Work out the finished part from the listing and answer in its coordinate system (mm). Face numbers are marked on the shaded views. A direction names the side the tool comes from. Round coordinates to 2 decimals unless told otherwise and drop trailing zeros. Order: outer loops, then holes, each group sorted by start corner. A loop starts at its lowest first (then second) coordinate and runs counter-clockwise, first axis right, second up. Notation, with made-up numbers: M 16,-12.75 L 46,-12.75 A21 cw 46,4.25 Z; hole C 18,-25.5 d10. An arc over 180 degrees is marked long. Return JSON: item names as keys, results as strings.
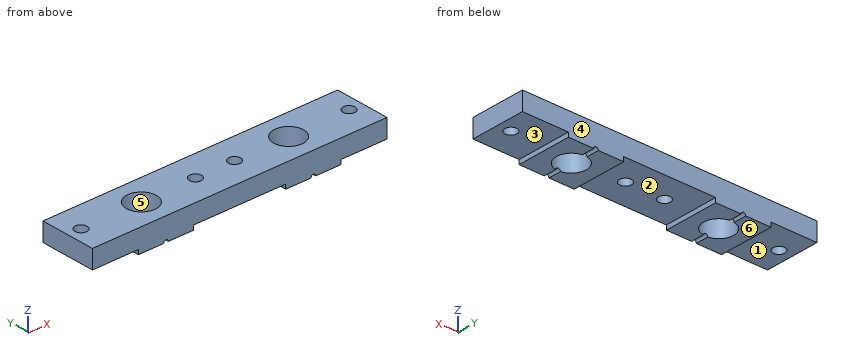
from build123d import *

# Parameters (mm, degrees)
SKETCH1_W                        = 101.6
SKETCH1_H                        = 19.05
EXTRUDE1_DEPTH                   = 7.9248
F_13_32_0_40625_DIAMETER_HOLE1_D = 10.31875
F_8_32_TAPPED_HOLE1_D            = 4.1656
SKETCH9_W                        = 31.75
SKETCH9_H                        = 19.05
SKETCH9_W_2                      = 15.875
EXTRUDE3_DEPTH                   = 1.524
F_1_16_0_0625_DIAMETER_HOLE1_D   = 1.5875


with BuildPart() as part:
    # Sketch1 → Extrude1 (new body)
    with BuildSketch(Plane.XY):
        Rectangle(SKETCH1_W, SKETCH1_H)
    extrude(amount=EXTRUDE1_DEPTH)

    # 13/32 (0.40625) Diameter Hole1 (through all)
    with Locations(Plane(origin=(0, 0, 0), x_dir=(-1, 0, 0), z_dir=(0, 0, -1))):
        with Locations((25.4, 0), (-25.4, 0)):
            Hole(F_13_32_0_40625_DIAMETER_HOLE1_D / 2)

    # #8-32 Tapped Hole1 (through all)
    with Locations(Plane.XY.offset(7.9248)):
        with Locations((-46.228, 0), (-6.731, 0), (6.731, 0), (46.228, 0)):
            Hole(F_8_32_TAPPED_HOLE1_D / 2)

    # Sketch9 → Extrude3 (cut)
    with BuildSketch(Plane(origin=(0, 0, 0), x_dir=(-1, 0, 0), z_dir=(0, 0, -1))):
        Rectangle(SKETCH9_W, SKETCH9_H)
        with Locations((-42.8625, 0)):
            Rectangle(SKETCH9_W_2, SKETCH9_H)
        with Locations((42.8625, 0)):
            Rectangle(SKETCH9_W_2, SKETCH9_H)
    extrude(amount=-EXTRUDE3_DEPTH, mode=Mode.SUBTRACT)

    # 1/16 (0.0625) Diameter Hole1 (through all)
    with Locations(Plane(origin=(0, 9.525, 0), x_dir=(-1, 0, 0), z_dir=(0, 1, 0))):
        with Locations((-25.4, 0), (25.4, 0)):
            Hole(F_1_16_0_0625_DIAMETER_HOLE1_D / 2)


solid = part.part
Item 1: Consider line 1 along Y through (x, z) = (-25, 1.75) (3 decimals); line 2 along X through (y, z) = (-3.5, 5); line 3 along X through (y, z) = (-4.5, 4.25). Determine where each line is inside the solid, lowest interval first. Write a range as [from, to].
Output:
{"line 1": "y = [-9.525, -5.144], [5.144, 9.525]", "line 2": "x = [-50.8, -29.19], [-21.61, 21.61], [29.19, 50.8]", "line 3": "x = [-50.8, -27.92], [-22.88, 22.88], [27.92, 50.8]"}
Item 2: Which of the six approach directions +Z, -Z, +X, -X, +Y, -Y give full straight-line access (tool end or side, diameter ignored) to the marked faces 1, 2 and 3?
Output:
{"face 1": "-Z, -X, +Y, -Y", "face 2": "-Z, +Y, -Y", "face 3": "-Z, +X, +Y, -Y"}
Item 3: Find section D-D (y = 3.5). Determine the outline of the cut face in (x, z) (3 decimals), plus the area to 3 significant figures.
Output:
{"outline": "M -50.8,1.524 L -34.925,1.524 L -34.925,0 L -29.191,0 L -29.191,7.925 L -50.8,7.925 Z; M -21.609,0 L -15.875,0 L -15.875,1.524 L 15.875,1.524 L 15.875,0 L 21.609,0 L 21.609,7.925 L -21.609,7.925 Z; M 29.191,0 L 34.925,0 L 34.925,1.524 L 50.8,1.524 L 50.8,7.925 L 29.191,7.925 Z", "area": "588 mm^2"}
Item 4: Find section A-A (z = 4.5). Determine the outline of the cut face in (x, y) (3 decimals), plus the area to 3 significant figures.
Output:
{"outline": "M -50.8,-9.525 L 50.8,-9.525 L 50.8,9.525 L -50.8,9.525 Z; hole C -46.228,0 d4.166; hole C -25.4,0 d10.319; hole C -6.731,0 d4.166; hole C 6.731,0 d4.166; hole C 25.4,0 d10.319; hole C 46.228,0 d4.166", "area": "1,710 mm^2"}
Item 5: The mould has two halves that part along Y. Classify the marked faces 4, 5 and 6: pulls with the +Y half, pulls with the -Y half, needs draft (parallel to the pull), parting line crosses it, or undercut.
Output:
{"face 4": "pulls with the +Y half", "face 5": "undercut", "face 6": "needs draft"}
Item 6: Each of these flat-tipped pins is pushed along its axis until it touches: pin 1 (5 mm diameter, centred on x = -45.5, y = 0, fed in from -Z); pin 2 (3.5 mm diameter, centred on x = -46.228, y = 0, fed in from -Z); pin 3 (0.5 mm diameter, centred on y = -0.5, z = 1, fed in from -X) (3 decimals); pin 4 (6.5 mm diameter, centred on x = 46.228, y = 0, fed in from +Z). Where does it stop, or does it pass through?
Output:
{"pin 1": "stops at z = 1.52", "pin 2": "passes through", "pin 3": "stops at x = -34.925", "pin 4": "stops at z = 7.92"}
Item 7: Find section C-C (x = 22). Determine the outline of the cut face in (y, z) (3 decimals), plus the area to 3 significant figures.
Output:
{"outline": "M -9.525,0 L -3.881,0 L -3.881,7.925 L -9.525,7.925 Z; M 3.881,0 L 9.525,0 L 9.525,7.925 L 3.881,7.925 Z", "area": "89.5 mm^2"}
Item 8: Find section B-B (y = -6.25). Determine the outline of the cut face in (x, z) (1 decimal), plus the area to 3 significant figures.
Output:
{"outline": "M -50.8,1.5 L -34.9,1.5 L -34.9,0 L -26.2,0 A0.8 cw -24.6,0 L -15.9,0 L -15.9,1.5 L 15.9,1.5 L 15.9,0 L 24.6,0 A0.8 cw 26.2,0 L 34.9,0 L 34.9,1.5 L 50.8,1.5 L 50.8,7.9 L -50.8,7.9 Z", "area": "706 mm^2"}
